```python
from build123d import *

# Parameters (mm, degrees)
SKETCH2_W           = 100
SKETCH2_H           = 100
BOSS_EXTRUDE1_DEPTH = 200
SHELL3_T            = -5
SKETCH3_W           = 90
SKETCH3_H           = 5
BOSS_EXTRUDE2_DEPTH = 85
SKETCH4_R           = 10
SKETCH4_R_2         = 2.5
BOSS_EXTRUDE3_DEPTH = 20
SKETCH5_R           = 10
SKETCH5_R_2         = 2.5
BOSS_EXTRUDE4_DEPTH = 20
SKETCH7_W           = 90
SKETCH7_H           = 5
CUT_EXTRUDE1_DEPTH  = 5


with BuildPart() as part:
    # Sketch2 → Boss-Extrude1 (new body)
    with BuildSketch(Plane(origin=(0, 0, 0), x_dir=(1, 0, 0), z_dir=(0, 1, 0))):
        with Locations((50, -50)):
            Rectangle(SKETCH2_W, SKETCH2_H)
    extrude(amount=BOSS_EXTRUDE1_DEPTH)

    # Shell3
    shell3_openings = [part.faces().sort_by_distance(p)[0] for p in [
        (50, 100, 100),
    ]]
    offset(amount=SHELL3_T, openings=shell3_openings, kind=Kind.INTERSECTION)

    # Sketch3 → Boss-Extrude2 (add)
    with BuildSketch(Plane.XY.offset(5)):
        with Locations((50, 57.5)):
            Rectangle(SKETCH3_W, SKETCH3_H)
        with Locations((50, 142.5)):
            Rectangle(SKETCH3_W, SKETCH3_H)
    extrude(amount=BOSS_EXTRUDE2_DEPTH)

    # Sketch4 → Boss-Extrude3 (add)
    with BuildSketch(Plane(origin=(100, 0, 0), x_dir=(0, 0, -1), z_dir=(1, 0, 0))):
        with Locations((-50, 100)):
            Circle(SKETCH4_R)
        with Locations((-50, 100)):
            Circle(SKETCH4_R_2, mode=Mode.SUBTRACT)
    extrude(amount=BOSS_EXTRUDE3_DEPTH)

    # Sketch5 → Boss-Extrude4 (add)
    with BuildSketch(Plane.ZY):
        with Locations((50, 100)):
            Circle(SKETCH5_R)
        with Locations((50, 100)):
            Circle(SKETCH5_R_2, mode=Mode.SUBTRACT)
    extrude(amount=BOSS_EXTRUDE4_DEPTH)

    # Sketch7 → Cut-Extrude1 (cut)
    with BuildSketch(Plane.XY.offset(100)):
        Polygon((95, 200), (0, 200), (0, 195), (5, 195), (95, 195), align=None)
        Polygon((100, 200), (95, 200), (95, 195), (95, 5), (95, 0), (100, 0), align=None)
        Polygon((5, 195), (0, 195), (0, 0), (5, 0), (5, 5), align=None)
        with Locations((50, 2.5)):
            Rectangle(SKETCH7_W, SKETCH7_H)
    extrude(amount=-CUT_EXTRUDE1_DEPTH, mode=Mode.SUBTRACT)


solid = part.part
```
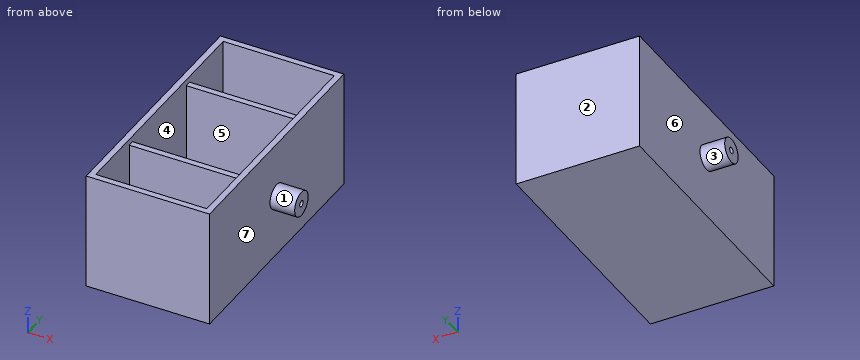
Check sheet for the modelled part. Datum: model origin and axes. Units: mm. Face numbers are marked on the shaded views. A direction names the side the tool comes from. Round coordinates to 2 decimals unless told otherwise and drop trailing zeros. Order: outer loops, then holes, each group sorted by start corner. A loop starts at its lowest first (then second) coordinate and runs counter-clockwise, first axis right, second up.
1) Go/stop test with flat-tipped pins: pin 1 Ø6 at (y, z) = (152.5, 61.5) entering from +X; pin 2 Ø4 at (x, y) = (84, 158) entering from +Z; pin 3 Ø1.5 at (x, y) = (39, 56.5) entering from +Z. Record where each tip stops, or that it passes through.
2) Scan lines: line 1 (Y direction, x = 84, z = 27); line 2 (X direction, y = 27.5, z = 91.5); line 3 (Y direction, x = 109.5, z = 50). Record each from-to range of solid material in increasing order.
3) Section check D-D (z = 14). Record the boundary of the cut face in (x, y).
4) Section check B-B (y = 100). Record the boundary of the cut face in (x, z), and give its area (3 significant figures).
5) Section check C-C (x = 35). Record the boundary of the cut face in (y, z).
6) Section check A-A (z = 50). Give the number of separate pieces and of enclosed holes in the cut face, and give its area (3 significant figures).
7) Mould release check, pull along X, two halves, no side actions. Record for the marked faces 5, 6 and 7: +X half, -X half, draft (parallel to the pull), parting line (faces both ways), or undercut.
8) Tool access check on the marked faces 1, 2, 3 and 4. Record the directions out of +Z, -Z, +X, -X, +Y, -Y that give a thin tool (end or side, any length) a straight path to the whole face; none if there is none.
Result:
1. pin 1: stops at x = 100
1. pin 2: stops at z = 5
1. pin 3: stops at z = 90
2. line 1: y = 0 to 5, 55 to 60, 140 to 145, 195 to 200
2. line 2: x = 0 to 5, 95 to 100
2. line 3: y = 90 to 97.5, 102.5 to 110
3. outline: (0, 0) - (100, 0) - (100, 200) - (0, 200) - close; hole (5, 5) - (95, 5) - (95, 55) - (5, 55) - close; hole (5, 60) - (95, 60) - (95, 140) - (5, 140) - close; hole (5, 145) - (95, 145) - (95, 195) - (5, 195) - close
4. outline: (-20, 40) - (0, 40) - (0, 0) - (100, 0) - (100, 40) - (120, 40) - (120, 47.5) - (100, 47.5) - (100, 52.5) - (120, 52.5) - (120, 60) - (100, 60) - (100, 95) - (95, 95) - (95, 5) - (5, 5) - (5, 95) - (0, 95) - (0, 60) - (-20, 60) - (-20, 52.5) - (0, 52.5) - (0, 47.5) - (-20, 47.5) - close
4. area: 2,000 mm2
5. outline: (0, 0) - (200, 0) - (200, 95) - (195, 95) - (195, 5) - (145, 5) - (145, 90) - (140, 90) - (140, 5) - (60, 5) - (60, 90) - (55, 90) - (55, 5) - (5, 5) - (5, 95) - (0, 95) - close
6. separate pieces: 1
6. enclosed holes: 3
6. area: 4,400 mm2
7. face 5: undercut
7. face 6: -X half
7. face 7: +X half
8. face 1: +X
8. face 2: +Z, -Z, +X, -X, +Y
8. face 3: -X
8. face 4: +Z
